For this review, take the finished solid that the model builds, in its own axes (mm). Round coordinates to 2 decimals unless told otherwise and drop trailing zeros. Order: outer loops, then holes, each group sorted by start corner. A loop starts at its lowest first (then second) coordinate and runs counter-clockwise, first axis right, second up. Notation, with made-up numbers: M 20.25,-2 L 70.25,-2 A25 ccw 70.25,22 Z; hole C -6.5,16 d9. An arc over 180 degrees is marked long. Use a Markdown table: item, result.
from build123d import *

# Parameters (mm, degrees)
PAD015_DEPTH                        = 3
SKETCH054_R                         = 1.65
POCKET018_DEPTH                     = 358.938883
POCKET018_DEPTH_BACK                = 361.938883
BODY001003005003004_PLACEMENT_ANGLE = 60


with BuildPart() as part:
    # Sketch053 → Pad015 (new body)
    with BuildSketch(Plane.XY):
        with BuildLine():
            ThreePointArc((152.005097, 113.785532), (84.992984, 169.790723), (0, 189.875477))
            Line((0, 189.875477), (0, 196.875477))
            ThreePointArc((157.608957, 117.98038), (88.126358, 176.050273), (0, 196.875477))
            ThreePointArc((152.005097, 113.785532), (156.904451, 113.081026), (157.608957, 117.98038))
        make_face()
    pad015 = extrude(amount=PAD015_DEPTH)

    # Sketch054 → Pocket018 (cut, two sides)
    with BuildSketch(Plane.XY) as pocket018_sk:
        with Locations((150.82443, 121.020933)):
            Circle(SKETCH054_R)
        with BuildLine():
            ThreePointArc((0, 191.725477), (1.65, 193.375477), (0, 195.025477))
            Line((0, 191.725477), (0, 195.025477))
        make_face()
    pocket018 = extrude(amount=-POCKET018_DEPTH, mode=Mode.SUBTRACT) + extrude(pocket018_sk.sketch, amount=POCKET018_DEPTH_BACK, mode=Mode.SUBTRACT)

    # Mirrored020: Pad015, Pocket018 across Sketch053 V_Axis
    add(pad015.mirror(Plane(origin=(0, 0, 0), x_dir=(0, 0, 1), z_dir=(1, 0, 0))))
    add(pocket018.mirror(Plane(origin=(0, 0, 0), x_dir=(0, 0, 1), z_dir=(1, 0, 0))), mode=Mode.SUBTRACT)


with BuildPart() as part_1:
    # Body001003005003004 placement: moved
    add(part.part.rotate(Axis((0, 0, 0), (0, 0, 1)), BODY001003005003004_PLACEMENT_ANGLE))


solid = part_1.part
Q1. Add section C-C (x = -69.5). Write out the cut boundary in (y, z), then the cut area to 3 significant figures.
Determined:
| item | result |
|---|---|
| outline | M 176.7,0 L 184.2,0 L 184.2,3 L 176.7,3 Z |
| area | 22.5 mm^2 |
Q2. Wall thickness on line 1 along Y through (x, z) = (-175.5, 2.4); line 2 along Y through (x, z) = (-29, 2.2); line 3 along Y through (x, z) = (-110, 2.5): over which ranges is each line inside the solid? List them lowest first. Write a range as [from, to].
Determined:
| item | result |
|---|---|
| line 1 | y = [-78.8, -72.47], [72.47, 89.22] |
| line 2 | y = [187.65, 189.53], [192.73, 194.73] |
| line 3 | y = [154.77, 163.28] |
Q3. Add section B-B (y = 24). Write out the cut boundary in (x, z), then the cut area to 3 significant figures.
Determined:
| item | result |
|---|---|
| outline | M -195.41,0 L -188.35,0 L -188.35,3 L -195.41,3 Z |
| area | 21.2 mm^2 |
Q4. Add section A-A (z = 2.45). Write out the cut boundary in (x, y), then the cut area to 3 significant figures.
Determined:
| item | result |
|---|---|
| outline | M -180.98,-77.5 A3.5 ccw -174.54,-74.75 A189.88 cw -164.44,94.94 A189.88 cw -22.54,188.53 A3.5 ccw -23.37,195.48 A196.88 ccw -170.5,98.44 A196.88 ccw Z; hole C -180.22,-70.11 d3.3; hole C -167.47,96.69 d3.3; hole C -29.39,191.13 d3.3 |
| area | 2,530 mm^2 |
